Autodesk Inventor part; units mm, degrees
ref_plane "YZ Plane" through (0, 0, 0) normal (1, 0, 0) x (0, 1, 0)
ref_plane "XZ Plane" through (0, 0, 0) normal (0, 1, 0) x (-1, 0, 0)
ref_plane "XY Plane" through (0, 0, 0) normal (0, 0, 1) x (1, 0, 0)
sketch "Sketch1" plane through (0, 0, 0) normal (0, 1, 0) x (-1, 0, 0)
  circle A0 centre (0, 0) radius 15
  circle A1 centre (0, 0) radius 8.5
  circle A2 centre (15, 0) radius 4
  circle A3 centre (-15, 0) radius 4
  line L0 (10.6066, -10.6066) -> (17.9306, -2.7224)
  line L1 (-10.6066, -10.6066) -> (-17.9306, -2.7224)
  line L2 (10.6066, 10.6066) -> (17.9306, 2.7224)
  line L3 (-10.6066, 10.6066) -> (-17.9306, 2.7224)
  line L4 (16.6, -2.7713) -> (13.4, -2.7713)
  line L5 (13.4, -2.7713) -> (11.8, 0)
  line L6 (11.8, 0) -> (13.4, 2.7713)
  line L7 (13.4, 2.7713) -> (16.6, 2.7713)
  line L8 (16.6, 2.7713) -> (18.2, 0)
  line L9 (18.2, 0) -> (16.6, -2.7713)
  line L10 (15, -2.7713) -> (15, 2.7713)
  line L11 (11.8, 0) -> (15, 0)
  line L12 (-13.4, -2.7713) -> (-16.6, -2.7713)
  line L13 (-16.6, -2.7713) -> (-18.2, 0)
  line L14 (-18.2, 0) -> (-16.6, 2.7713)
  line L15 (-16.6, 2.7713) -> (-13.4, 2.7713)
  line L16 (-13.4, 2.7713) -> (-11.8, 0)
  line L17 (-11.8, 0) -> (-13.4, -2.7713)
  line L18 (-15, -2.7713) -> (-15, 2.7713)
  line L19 (-18.2, 0) -> (-15, 0)
  circle A4 centre (0, 0) radius 6
  circle A5 centre (0, -6) radius 1.2
  circle A6 centre (-6, 0) radius 1.2
  circle A7 centre (0, 6) radius 1.2
  circle A8 centre (6, 0) radius 1.2
  circle A9 centre (15, 0) radius 1.65
  circle A10 centre (-15, 0) radius 1.65
  point P0 (-11.3582, -9.7975)
  point P1 (11.3582, -9.7975)
  point P2 (11.3582, 9.7976)
  point P3 (-11.3582, 9.7976)
  dimension "d20" = 8
  dimension "d22" = 3.2
  dimension "d27" = 3.2
  dimension "d28" = 3.2
  dimension "d29" = 120
  dimension "d30" = 3.2
  dimension "d31" = 120
  dimension "d34" = 12
  dimension "d35" = 2.4
  dimension "d36" = 2.4
  dimension "d37" = 2.4
  dimension "d38" = 2.4
  dimension "d43" = 3.3
  dimension "d44" = 3.3
extrude "Extrusion1" add sketch "Sketch1" along normal blind 10 contours L2 A0 A2 L0 L1 A3 L3 | A0 L2 | L3 A0 | L2 A2 A0 | A0 A3 L3 | A2 A0 L4 L9 L8 L7 | A0 L7 L6 L5 L4 A2 | A3 A0 L12 L17 L16 L15 | A0 L15 L14 L13 L12 A3 | L7 L10 A9 A0 | A0 A9 L11 L6 L7 | A2 L0 A0 | L15 L16 L17 L12 A0 A10 | A0 A10 L18 L15 | A3 A0 L1 | A9 L10 A0 | A0 L11 A9 | L7 L8 L9 L4 L10 A9 | A0 L0 | L4 L5 L11 A9 A0 | A0 A9 L10 L4 | A10 A0 | A0 L18 A10 | L18 A10 L19 L14 L15 | L1 A0 | L10 A9 A0 | L10 A9 | A0 A9 L11 | A0 A10 L18 | L19 A10 L18 | L18 A10 L19 | L12 L18 A10 A0 | L18 L12 L13 L19 A10 | A1 | A4 A8 | A4 A8 | A8 A4 A5 A6 A7 | A7 A4 | A4 A7 | A5 A4 | A4 A5 | A6 A4 | A4 A6
extrude "Extrusion2" cut sketch "Sketch1" along normal blind 2.5 contours L7 L10 A9 A0 | A0 A9 L11 L6 L7 | L15 L16 L17 L12 A0 A10 | A0 A10 L18 L15 | A9 L10 A0 | A0 L11 A9 | L7 L8 L9 L4 L10 A9 | L4 L5 L11 A9 A0 | A0 A9 L10 L4 | A10 A0 | A0 L18 A10 | L18 A10 L19 L14 L15 | L10 A9 A0 | L10 A9 | A0 A9 L11 | A0 A10 L18 | L19 A10 L18 | L18 A10 L19 | L12 L18 A10 A0 | L18 L12 L13 L19 A10 | A1 | A4 A8 | A4 A8 | A8 A4 A5 A6 A7 | A7 A4 | A4 A7 | A5 A4 | A4 A5 | A6 A4 | A4 A6
extrude "Extrusion3" cut sketch "Sketch1" along normal blind 10 contours A9 L10 A0 | A0 L11 A9 | A10 A0 | A0 L18 A10 | L10 A9 A0 | L10 A9 | A0 A9 L11 | A0 A10 L18 | L19 A10 L18 | L18 A10 L19 | A4 A8 | A4 A8 | A7 A4 | A4 A7 | A5 A4 | A4 A5 | A6 A4 | A4 A6
fillet "Fillet1" radius 0.3 16 edges at (0, 0, -15) (-19, 0, 0) (-14.6444, 0, 6.26) (-14.6444, 0, -6.26) (0, 0, 15) (19, 0, 0) (14.6444, 0, -6.26) (14.6444, 0, 6.26) (-19, 10, 0) (-14.6444, 10, 6.26) (-14.6444, 10, -6.26) (0, 10, -15) (0, 10, 15) (19, 10, 0) (14.6444, 10, 6.26) (14.6444, 10, -6.26)
sketch "Sketch2" plane through (0, 10, 0) normal (0, 1, 0) x (1, 0, 0)
  circle A0 centre (-6, 0) radius 1.2
  circle A1 centre (-6, 0) radius 2
  circle A2 centre (0, 6) radius 1.2
  circle A3 centre (0, 6) radius 2
  circle A4 centre (6, 0) radius 1.2
  circle A5 centre (6, 0) radius 2
  circle A6 centre (0, -6) radius 1.2
  circle A7 centre (0, -6) radius 2
  point P0 (0, 0)
  dimension "d48" = 4
  dimension "d49" = 4
  dimension "d50" = 4
  dimension "d51" = 4
extrude "Extrusion5" cut sketch "Sketch2" against normal blind 2 contours A0 | A1 | A2 | A3 | A4 | A5 | A6 | A7
properties part number "neck"
For this review, take the finished solid that the model builds, in its own axes (mm). A direction names the side the tool comes from. Round coordinates to 2 decimals unless told otherwise and drop trailing zeros. Write each loop counter-clockwise with the first axis right and the second up, starting at its lowest first coordinate (ties: lowest second). Pieces come first, ordered by that corner, then holes. Notation, with made-up numbers: (41.25, -5) - (63.25, -5) arc R23 ccw to (63.25, 16) - close; hole circle Ø2 at (50, 72). An arc over 180 degrees is marked (long way). Answer as a JSON object with one key per item and string values.
1. We need section B-B on y = 4. Give the boundary of the cut face in (x, z).
Response values:
{"outline": "(-17.93, -2.72) - (-11.36, -9.8) arc R15 ccw to (11.36, -9.8) - (17.93, -2.72) arc R4 ccw to (17.93, 2.72) - (11.36, 9.8) arc R15 ccw to (-11.36, 9.8) - (-17.93, 2.72) arc R4 ccw to start; hole circle Ø3.3 at (-15, 0); hole circle Ø2.4 at (-6, 0); hole circle Ø2.4 at (0, -6); hole circle Ø2.4 at (0, 6); hole circle Ø2.4 at (6, 0); hole circle Ø3.3 at (15, 0)"}
2. Draft analysis for pull direction Z (two halves, no side actions). For faces 3 (the face through (-14.532, 9.914, 6.248)), 4 (the face through (-15, 1, 2.771)), 5 (the face through (14.6, 4.93, -6.31)), state which applies: +Z half, -Z half, draft (parallel to the pull), parting line (faces both ways), or undercut.
Response values:
{"face 3": "+Z half", "face 4": "undercut", "face 5": "-Z half"}
3. We need section A-A on x = 0. Give the boundary of the cut face in (y, z), then the cut area to 3 significant figures.
Response values:
{"outline": "(0, -14.7) arc R0.3 ccw to (0.3, -15) - (9.7, -15) arc R0.3 ccw to (10, -14.7) - (10, -8) - (8, -8) - (8, -7.2) - (2.5, -7.2) - (2.5, -8.5) - (0, -8.5) - close; (0, 8.5) - (2.5, 8.5) - (2.5, 7.2) - (8, 7.2) - (8, 8) - (10, 8) - (10, 14.7) arc R0.3 ccw to (9.7, 15) - (0.3, 15) arc R0.3 ccw to (0, 14.7) - close; (2.5, -4.8) - (8, -4.8) - (8, -4) - (10, -4) - (10, 4) - (8, 4) - (8, 4.8) - (2.5, 4.8) - close", "area": "215 mm2"}
4. To check wall thickness, follow line 1 along X through (y, z) = (3, -0.5); line 2 along Z through (x, y) = (0.5, 8.75); line 3 along Y through (x, z) = (-7.5, -3). State the ranges of each line that lie inside material, in increasing order.
Response values:
{"line 1": "x = -18.97 to -16.57, -13.43 to -7.09, -4.91 to 4.91, 7.09 to 13.43, 16.57 to 18.97", "line 2": "z = -14.99 to -7.94, -4.06 to 4.06, 7.94 to 14.99", "line 3": "y = 2.5 to 10"}
5. We need section D-D on z = 0.5. Count the separate pieces of the cut face and the enclosed holes in it, then the cut area to 3 significant figures.
Response values:
{"separate pieces": "5", "enclosed holes": "0", "area": "221 mm2"}
6. We need section C-C on y = 1. Give the boundary of the cut face in (x, z), then the cut area to 3 significant figures.
Response values:
{"outline": "(-17.93, -2.72) - (-11.36, -9.8) arc R15 ccw to (11.36, -9.8) - (17.93, -2.72) arc R4 ccw to (17.93, 2.72) - (11.36, 9.8) arc R15 ccw to (-11.36, 9.8) - (-17.93, 2.72) arc R4 ccw to start; hole (-18.2, 0) - (-16.6, -2.77) - (-13.4, -2.77) - (-11.8, 0) - (-13.4, 2.77) - (-16.6, 2.77) - close; hole circle Ø17 at (0, 0); hole (11.8, 0) - (13.4, -2.77) - (16.6, -2.77) - (18.2, 0) - (16.6, 2.77) - (13.4, 2.77) - close", "area": "502 mm2"}
7. For pin 1 Ø2 at (x, y) = (-4, 5) entering from +Z; pin 2 Ø3 at (x, z) = (6, 0) entering from -Y; pin 3 Ø3 at (x, y) = (-15, 0.5) entering from +Z, all flat-tipped, find the tip position at first contact; note any pin that passes through.
Response values:
{"pin 1": "stops at z = 14.7", "pin 2": "stops at y = 2.5", "pin 3": "stops at z = 7.49"}
8. Tool access review of faces 1 (the face through (-4.8, 5.21, -0.05)), 2 (the face through (-17.389, 1.232, 1.405)): name each direction out of +Z, -Z, +X, -X, +Y, -Y from which nothing blocks a thin tool from reaching the whole face with its end or side.
Response values:
{"face 1": "+Y, -Y", "face 2": "-Y"}
